The drawing under review shows one solid part. Ordinate dimensions are in mm from its lowest x, y, z. A direction names the side the tool comes from. Round coordinates to 2 decimals unless told otherwise and drop trailing zeros. Write each loop counter-clockwise with the first axis right and the second up, starting at its lowest first coordinate (ties: lowest second). Pieces come first, ordered by that corner, then holes. Notation, with made-up numbers: (7, 22.5) -> (19, 22.5) arc R19 ccw to (19, 37.5) -> close; hole circle Ø7 at (2, -15.75). An arc over 180 degrees is marked (long way). Write item = value, one per line. Start each with the question number.
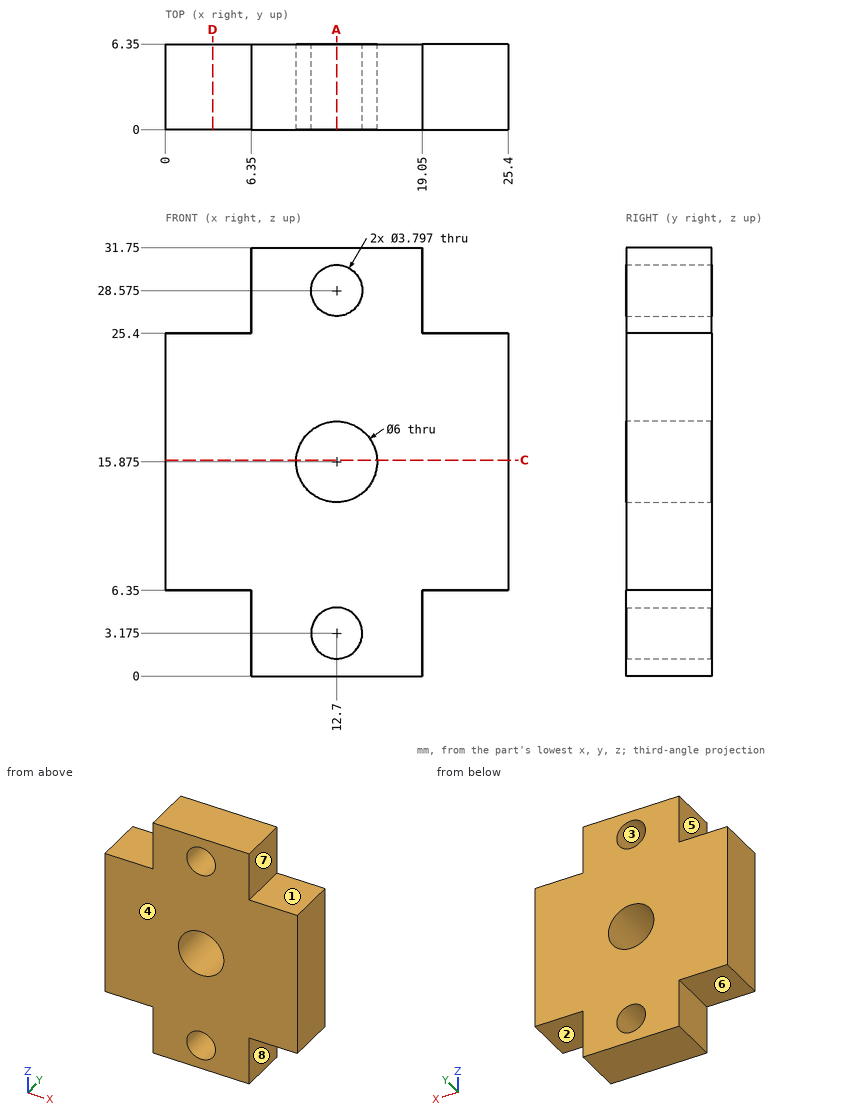
1. Draft analysis for pull direction Z (two halves, no side actions). For the marked faces 1, 2, 3 and 4, state which applies: +Z half, -Z half, draft (parallel to the pull), parting line (faces both ways), or undercut.
2. Consider section D-D, the plane x = 3.5. Give the boundary of the cut face in (y, z).
3. Consider section C-C, the plane z = 16. Give the boundary of the cut face in (x, y).
4. Consider section A-A, the plane x = 12.7. Give the number of separate pieces and of enclosed holes in the cut face, then the cut area to 3 significant figures.
5. Clearance check with flat-ended pins moving along their axes: pin 1 Ø1.9 at (x, y) = (3, 2.5) entering from -Z; pin 2 Ø1.9 at (y, z) = (2, 4) entering from +X; pin 3 Ø9.5 at (x, z) = (12.7, 15.875) entering from -Y; pin 4 Ø1.9 at (y, z) = (3.5, 29) entering from -X. State where each tip first meets the part, or that it passes through.
6. Machinability: for the marked faces 5, 6, 7 and 8, which of the approach directions +Z, -Z, +X, -X, +Y, -Y give a long, thin tool a straight path to every point of the face, cutting with its end or side? Answer none if there is none.
7. Wall thickness on L1, parallel to X at y = 4, z = 3; L2, parallel to X at y = 4.25, z = 16; L3, parallel to Z at x = 4.25, y = 2: over which ranges is each line inside the solid? List them lowest first. Write a range as from..to.
Outcome:
q1.face_1 = +Z half
q1.face_2 = -Z half
q1.face_3 = undercut
q1.face_4 = draft
q2.outline = (0, 6.35) -> (6.35, 6.35) -> (6.35, 25.4) -> (0, 25.4) -> close
q3.outline = (0, 0) -> (9.7, 0) -> (9.7, 6.35) -> (0, 6.35) -> close; (15.7, 0) -> (25.4, 0) -> (25.4, 6.35) -> (15.7, 6.35) -> close
q4.separate_pieces = 4
q4.enclosed_holes = 0
q4.area = 115 mm2
q5.pin_1 = 6.35
q5.pin_2 = 19.05
q5.pin_3 = 0
q5.pin_4 = 6.35
q6.face_5 = +Z, -X, +Y, -Y
q6.face_6 = -Z, -X, +Y, -Y
q6.face_7 = +Z, +X, +Y, -Y
q6.face_8 = -Z, +X, +Y, -Y
q7.L1 = 6.35..10.81, 14.59..19.05
q7.L2 = 0..9.7, 15.7..25.4
q7.L3 = 6.35..25.4
